Autodesk Inventor part; units mm, degrees
ref_plane "YZ Plane" through (0, 0, 0) normal (1, 0, 0) x (0, 1, 0)
ref_plane "XZ Plane" through (0, 0, 0) normal (0, 1, 0) x (-1, 0, 0)
ref_plane "XY Plane" through (0, 0, 0) normal (0, 0, 1) x (1, 0, 0)
sketch "Skizze2" plane through (0, 0, 0) normal (1, 0, 0) x (0, 1, 0)
  line L0 (0, 0) -> (15, 0)
  line L1 (15, 0) -> (15, 2)
  line L2 (15, 2) -> (2, 2)
  line L3 (2, 2) -> (2, 47)
  line L4 (2, 47) -> (0, 47)
  line L5 (0, 47) -> (0, 0)
  dimension "d0" = 2
  dimension "d2" = 45
  dimension "d3" = 2
  dimension "d4" = 90
  dimension "d5" = 15
extrude "Extrusion1" add sketch "Skizze2" against normal blind 20
sketch "Skizze3" plane through (0, 2, 2) normal (0, 0, 1) x (1, 0, 0)
  circle A0 centre (-10, 5.5) radius 1.6
  line L0 (0, 13) -> (0, 0)
  line L1 (0, 0) -> (-20, 0)
  line L2 (0, -2) -> (-20, -2)
  dimension "d8" = 3.2
  dimension "d9" = 10
  dimension "d17" = 7.5
extrude "Extrusion2" cut sketch "Skizze3" against normal through all
sketch "Skizze4" plane through (0, 2, 47) normal (0, 1, 0) x (1, 0, 0)
  line L0 (0, 0) -> (-20, 0)
  line L1 (0, -12.4844) -> (12.4058, -12.4844)
  line L2 (12.4058, -12.4844) -> (12.4058, -4.4844)
  line L3 (12.4058, -4.4844) -> (0, -4.4844)
  line L4 (0, -4.4844) -> (0, 0)
  line L5 (0, 0) -> (-20, 0)
  line L6 (-20, 47) -> (-20, 0)
  line L7 (-20, 0) -> (-20, -12.4844)
  line L8 (-20, -12.4844) -> (0, -12.4844)
  point P0 (0, 47)
  dimension "d13" = 8
extrude "Extrusion3" add sketch "Skizze4" against normal blind 2
sketch "Skizze5" plane through (-20, 2, 2) normal (0, 1, 0) x (1, 0, 0)
  circle A0 centre (25.895, -53.9844) radius 1.6
  circle A1 centre (15.895, -53.9844) radius 1.6
  line L0 (0, -57.4844) -> (32.4058, -57.4844)
  point P0 (20, 2)
  dimension "d18" = 3.2
  dimension "d19" = 3.2
  dimension "d20" = 10
  dimension "d21" = 3.5
  dimension "d22" = 3.5
extrude "Extrusion4" cut sketch "Skizze5" against normal through all
fillet "Rundung1" radius 2 2 edges at (-10, 2, 2) (-10, 0, 0)
fillet "Rundung2" radius 0.8 6 edges at (-3.7971, 2, 59.4844) (-3.7971, 0, 59.4844) (6.2029, 2, 51.4844) (-10, 15, 2) (-10, 15, 0) (6.2029, 0, 51.4844)
properties part number "X-Endstop holder mount" material "ABS-Kunststoff"
For this review, take the finished solid that the model builds, in its own axes (mm). A direction names the side the tool comes from. Coordinates: 2 decimals unless noted, no trailing zeros. Write each loop counter-clockwise with the first axis right and the second up, starting at its lowest first coordinate (ties: lowest second). Pieces come first, ordered by that corner, then holes.
(1) Add section B-B on y = 7.5. Give the boundary of the cut face in (x, z).
(2) Tool access review of faces 4 (the face through (-9.9, 9.4, 0)), 5 (the face through (-10, 10, 2)): name each direction out of +Z, -Z, +X, -X, +Y, -Y from which nothing blocks a thin tool from reaching the whole face with its end or side.
(3) Add section D-D on z = 12.5. Give the boundary of the cut face in (x, y), then the cut area to 3 significant figures.
(4) For pin 1 Ø4 at (x, y) = (-11.5, 8) entering from -Z; pin 2 Ø5 at (x, z) = (-12, 43) entering from +Y, all flat-tipped, find the tip position at first contact; note any pin that passes through.
(5) Add section A-A on x = -10. Give the boundary of the cut face in (y, z).
(6) The part is to be moulded in two halves that separate along X. For faces 1 (the face through (-11.27, 6.53, 1.01)), 2 (the face through (12.406, 1, 56)), 3 (the face through (-10.14, 0.6, 0.57)), say which applies: +X half, -X half, draft (parallel to the pull), parting line (faces both ways), or undercut.
(7) Add section C-C on x = -13.5. Give the boundary of the cut face in (y, z), then the cut area to 3 significant figures.
(8) Wall thickness on probe 1 along Y at (x, z) = (-14, 55.5); probe 2 along Y at (x, z) = (-10, 1.1): over which ranges is each line inside the solid? List them lowest first.
Answer sheet:
1. outline: (-20, 0) - (-11.6, 0) - (-11.6, 2) - (-20, 2) - close; (-8.4, 0) - (0, 0) - (0, 2) - (-8.4, 2) - close
2. face 4: -Z, +X, -X, +Y, -Y
2. face 5: +Z, +X, -X, +Y
3. outline: (-20, 0) - (0, 0) - (0, 2) - (-20, 2) - close
3. area: 40.0 mm2
4. pin 1: stops at z = 0
4. pin 2: stops at y = 2
5. outline: (0, 2) arc R2 ccw to (2, 0) - (5.9, 0) - (5.9, 2) - (4, 2) arc R2 cw to (2, 4) - (2, 58.68) arc R0.8 ccw to (1.2, 59.48) - (0.8, 59.48) arc R0.8 ccw to (0, 58.68) - close; (9.1, 0) - (14.2, 0) arc R0.8 ccw to (15, 0.8) - (15, 1.2) arc R0.8 ccw to (14.2, 2) - (9.1, 2) - close
6. face 1: undercut
6. face 2: +X half
6. face 3: draft
7. outline: (0, 2) arc R2 ccw to (2, 0) - (14.2, 0) arc R0.8 ccw to (15, 0.8) - (15, 1.2) arc R0.8 ccw to (14.2, 2) - (4, 2) arc R2 cw to (2, 4) - (2, 58.68) arc R0.8 ccw to (1.2, 59.48) - (0.8, 59.48) arc R0.8 ccw to (0, 58.68) - close
7. area: 144 mm2
8. probe 1: y = 0 to 2
8. probe 2: y = 0.21 to 5.9, 9.1 to 15
